Job drawing, mm, ordinate dimensions from the low corner. One solid piece. A direction names the side the tool comes from. Coordinates: 2 decimals unless noted, no trailing zeros. Loops run counter-clockwise (first coordinate to the right, second up) from the corner with the lowest first, then second, coordinate; pieces in that order, holes last. Notation, with made-up numbers: (86, -5) - (103, -5) arc R26 cw to (103, 31) - close; hole circle Ø11 at (81.5, -5). An arc over 180 degrees is marked (long way). Use a Markdown table: item, result. Add a question column.
1. Band-saw the part on D-D, the plane x = 11. Give the cut face in (y, z).
2. Band-saw the part on C-C, the plane z = 18.5. Give the cut face in (x, y).
3. Drop flat-ended pins along their axis: pin 1 (10 mm diameter, centred on x = 12, z = 27, fed in from -Y); pin 2 (5 mm diameter, centred on x = 16, y = 2.5, fed in from -Z) (1 decimal); pin 3 (7.5 mm diameter, centred on y = 8, z = 16.5, fed in from +X); pin 4 (2 mm diameter, centred on y = 10, z = 34.5, fed in from -X) (1 decimal). Give the stop position or say it passes through.
4. 3-axis set-ups, long thin cutter, end or side, ignore diameter. For the marked faces 4 and 5: which of +Z, -Z, +X, -X, +Y, -Y reach the whole face in a straight line?
5. Band-saw the part on A-A, the plane z = 35. Give the cut face in (x, y).
6. Pull direction X, two halves, no side cores. Call the marked faces 1, 2 and 3: pulls with the +X half, pulls with the -X half, needs draft (parallel to the pull), parting line crosses it, or undercut.
7. Wall check: probe 1 along X at (y, z) = (11, 40.5) (1 decimal); probe 2 along X at (y, z) = (8.25, 15.5) (1 decimal); probe 3 along Z at (x, y) = (18, 4.75) (1 decimal). Give the ranges that are in metal, low to high. Write a range as [from, to].
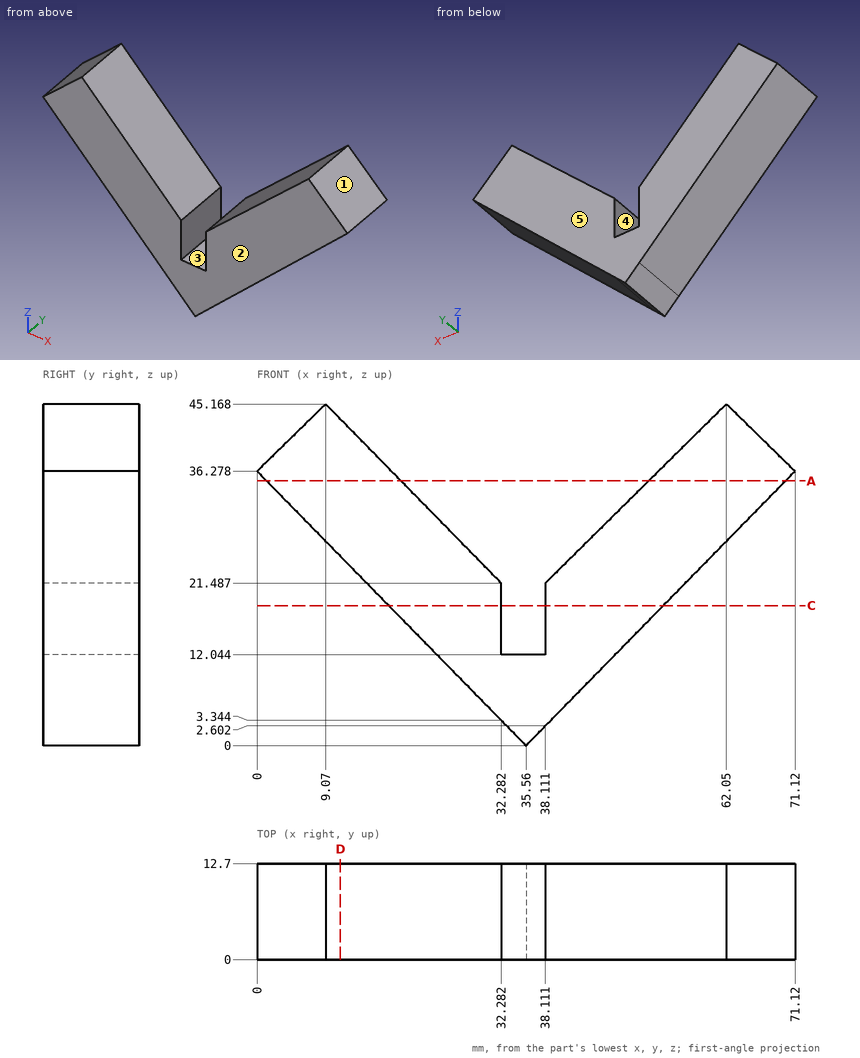
Geometry check:
| question | item | result |
|---|---|---|
| 1 | outline | (0, 25.06) - (12.7, 25.06) - (12.7, 43.2) - (0, 43.2) - close |
| 2 | outline | (17.43, 0) - (32.28, 0) - (32.28, 12.7) - (17.43, 12.7) - close; (38.11, 0) - (53.69, 0) - (53.69, 12.7) - (38.11, 12.7) - close |
| 3 | pin 1 | stops at y = 0 |
| 3 | pin 2 | stops at z = 17.4 |
| 3 | pin 3 | stops at x = 55.41 |
| 3 | pin 4 | stops at x = 0.8 |
| 4 | face 4 | +Z, +Y, -Y |
| 4 | face 5 | +Z, -Z, +X, -X, +Y |
| 5 | outline | (1.25, 0) - (19.04, 0) - (19.04, 12.7) - (1.25, 12.7) - close; (51.77, 0) - (69.87, 0) - (69.87, 12.7) - (51.77, 12.7) - close |
| 6 | face 1 | pulls with the +X half |
| 6 | face 2 | needs draft |
| 6 | face 3 | undercut |
| 7 | probe 1 | x = [4.3, 13.6], [57.3, 66.8] |
| 7 | probe 2 | x = [20.4, 32.3], [38.1, 50.8] |
| 7 | probe 3 | z = [17.9, 36.1] |
